Check sheet for the drawn part. Datum: minimum x, y, z corner. Units: mm. A direction names the side the tool comes from. Coordinates: 2 decimals unless noted, no trailing zeros. Loops run counter-clockwise (first coordinate to the right, second up) from the corner with the lowest first, then second, coordinate; pieces in that order, holes last. Notation, with made-up numbers: M 65,77 L 91,77 A15 ccw 91,86 Z; hole C 31,84 d7. An arc over 180 degrees is marked long. Answer in a Markdown table with one row per item. Add a question column.
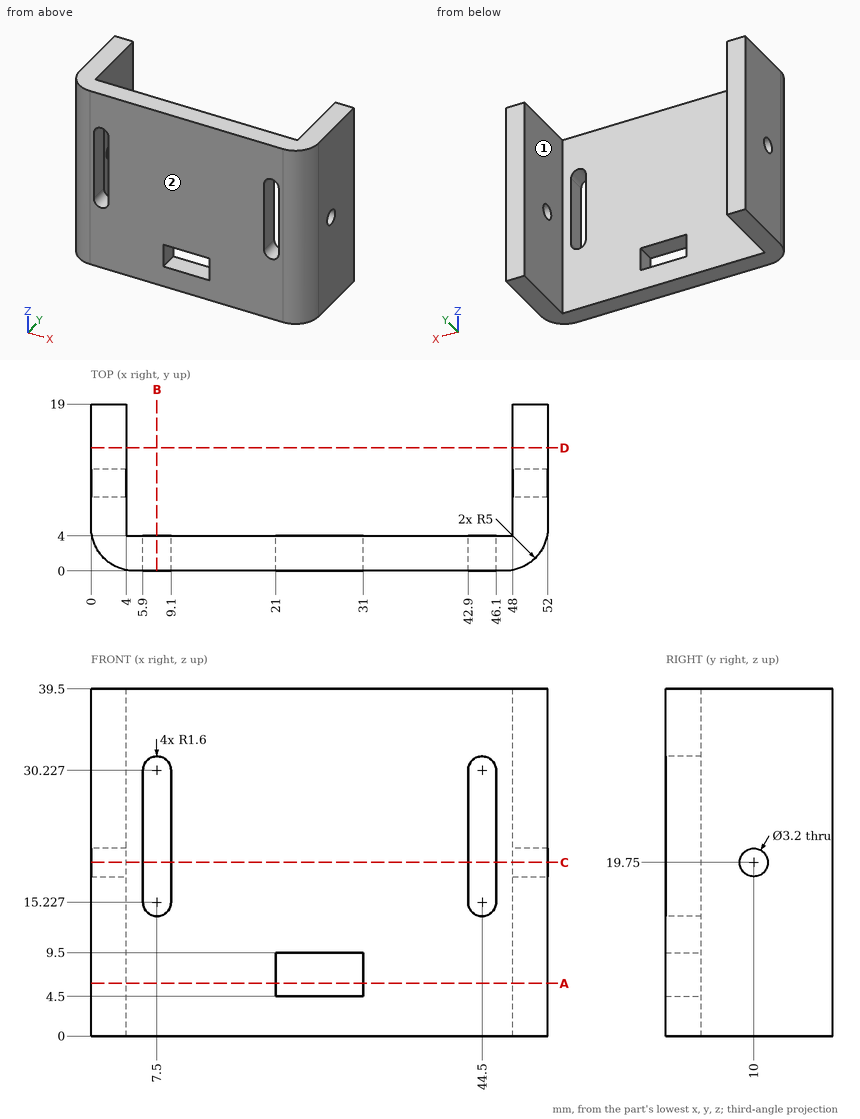
Q1. Cross-section at D-D (y = 14). Record the cut outline in (x, z).
Q2. Cross-section at A-A (z = 6). Record the cut outline in (x, y).
Q3. Cross-section at B-B (x = 7.5). Record the cut outline in (y, z), plus the area to 3 significant figures.
Q4. Access from +Z, -Z, +X, -X, +Y, -Y to the whole of each face (thin tool, end or side, straight path). Record for the marked faces 1 and 2.
Q5. Go/stop test with flat-tipped pins: pin 1 (10 mm diameter, centred on y = 10, z = 19, fed in from +X); pin 2 (1.9 mm diameter, centred on y = 10, z = 19.75, fed in from +X); pin 3 (1.2 mm diameter, centred on y = 2.5, z = 7, fed in from +X) (3 decimals); pin 4 (2 mm diameter, centred on y = 2.5, z = 23.5, fed in from -X). Record where each tip stops, or that it passes through.
Q6. Thickness scan on L1, parallel to X at y = 8.5, z = 10; L2, parallel to X at y = 1.25, z = 14.5 (1 decimal); L3, parallel to Z at x = 49.9, y = 10. Record the ranges inside material, lowest first.
Q7. Cross-section at C-C (z = 19.75). Record the cut outline in (x, y).
Answer key:
| question | item | result |
|---|---|---|
| 1 | outline | M 0,0 L 4,0 L 4,39.5 L 0,39.5 Z; M 48,0 L 52,0 L 52,39.5 L 48,39.5 Z |
| 2 | outline | M 0,5 A5 ccw 5,0 L 21,0 L 21,4 L 4,4 L 4,19 L 0,19 Z; M 31,0 L 47,0 A5 ccw 52,5 L 52,19 L 48,19 L 48,4 L 31,4 Z |
| 3 | outline | M 0,0 L 4,0 L 4,13.63 L 0,13.63 Z; M 0,31.83 L 4,31.83 L 4,39.5 L 0,39.5 Z |
| 3 | area | 85.2 mm^2 |
| 4 | face 1 | +Z, -Z, +Y |
| 4 | face 2 | +Z, -Z, +X, -X, -Y |
| 5 | pin 1 | x = 52 |
| 5 | pin 2 | through |
| 5 | pin 3 | x = 51.625 |
| 5 | pin 4 | x = 0.23 |
| 6 | L1 | 0 to 4, 48 to 52 |
| 6 | L2 | 1.7 to 6.1, 8.9 to 43.1, 45.9 to 50.3 |
| 6 | L3 | 0 to 18.15, 21.35 to 39.5 |
| 7 | outline | M 0,5 A5 ccw 5,0 L 5.9,0 L 5.9,4 L 4,4 L 4,8.4 L 0,8.4 Z; M 0,11.6 L 4,11.6 L 4,19 L 0,19 Z; M 9.1,0 L 42.9,0 L 42.9,4 L 9.1,4 Z; M 46.1,0 L 47,0 A5 ccw 52,5 L 52,8.4 L 48,8.4 L 48,4 L 46.1,4 Z; M 48,11.6 L 52,11.6 L 52,19 L 48,19 Z |
